Could you check a few things on this drawing? It's one solid part, dimensions in mm from its lowest x, y, z. A direction names the side the tool comes from. Round coordinates to 2 decimals unless told otherwise and drop trailing zeros. Order: outer loops, then holes, each group sorted by start corner. A loop starts at its lowest first (then second) coordinate and runs counter-clockwise, first axis right, second up. Notation, with made-up numbers: (1.25, 60) -> (51.25, 60) arc R9 cw to (51.25, 77) -> close; hole circle Ø2 at (45, 45). An arc over 180 degrees is marked (long way). Use a Markdown table: item, result. Add a question column.
(1) On a 3-axis mill with a long thin cutter (end or side, diameter ignored), from which of +Z, -Z, +X, -X, +Y, -Y can I reach the whole of each face in a straight line? I mean the marked faces 4, 5 and 6. Say none if no direction works.
(2) Thinking about a two-plate mould opening in Z: for the marked faces 1, 2 and 3, which applies, pulls with the +Z half, pulls with the -Z half, needs draft (parallel to the pull), parting line crosses it, or undercut?
(3) I want a section at C-C, the plane y = 34. Please give me the cut outline in (x, z), then the cut area to 3 significant figures.
(4) I want a section at B-B, the plane z = 2.5. Please give me the cut outline in (x, y) (3 decimals), then the cut area to 3 significant figures.
(5) I'm going to push flat-ended pins straight in: P1, Ø3, axis at y = 47, z = 3, coming from the -X side; P2, Ø1.8, axis at x = 89, z = 3, coming from the +Y side; P3, Ø3, axis at y = 39, z = 4, coming from the +X side. Where does each tip first touch, or does it pass through?
(6) If I drill on probe 1 along Y at (x, z) = (23, 0.3); probe 2 along X at (y, z) = (45, 2.5); probe 3 along X at (y, z) = (40, 5.35), over which ranges is the centre line in solid material (lowest first)?
(7) I want a section at A-A, the plane y = 42. Please give me the cut outline in (x, z) (3 decimals), then the cut area to 3 significant figures.
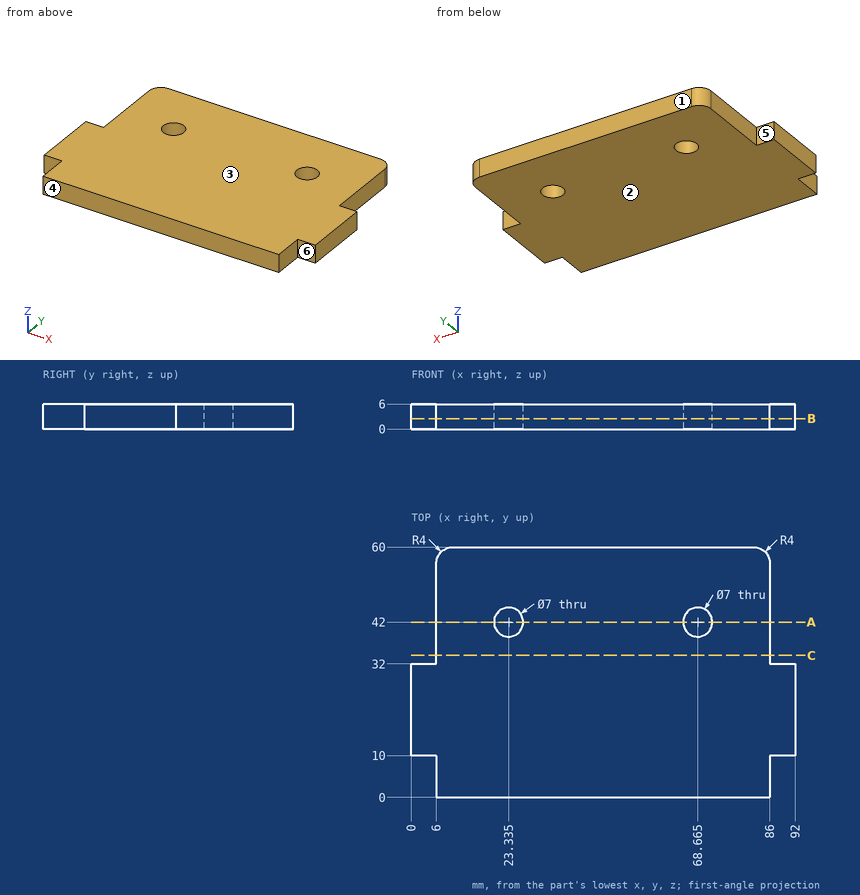
Taken from the geometry:
| question | item | result |
|---|---|---|
| 1 | face 4 | +Z, -Z, +X, -X, -Y |
| 1 | face 5 | +Z, -Z, -X, +Y |
| 1 | face 6 | +Z, -Z, +X, -Y |
| 2 | face 1 | needs draft |
| 2 | face 2 | pulls with the -Z half |
| 2 | face 3 | pulls with the +Z half |
| 3 | outline | (6, 0) -> (86, 0) -> (86, 6) -> (6, 6) -> close |
| 3 | area | 480 mm2 |
| 4 | outline | (0, 10) -> (6, 10) -> (6, 0) -> (86, 0) -> (86, 10) -> (92, 10) -> (92, 32) -> (86, 32) -> (86, 56) arc R4 ccw to (82, 60) -> (10, 60) arc R4 ccw to (6, 56) -> (6, 32) -> (0, 32) -> close; hole circle Ø7 at (23.335, 42); hole circle Ø7 at (68.665, 42) |
| 4 | area | 4,980 mm2 |
| 5 | P1 | stops at x = 6 |
| 5 | P2 | stops at y = 32 |
| 5 | P3 | stops at x = 86 |
| 6 | probe 1 | y = 0 to 38.52, 45.48 to 60 |
| 6 | probe 2 | x = 6 to 21.53, 25.14 to 66.86, 70.47 to 86 |
| 6 | probe 3 | x = 6 to 20.46, 26.21 to 65.79, 71.54 to 86 |
| 7 | outline | (6, 0) -> (19.835, 0) -> (19.835, 6) -> (6, 6) -> close; (26.835, 0) -> (65.165, 0) -> (65.165, 6) -> (26.835, 6) -> close; (72.165, 0) -> (86, 0) -> (86, 6) -> (72.165, 6) -> close |
| 7 | area | 396 mm2 |
